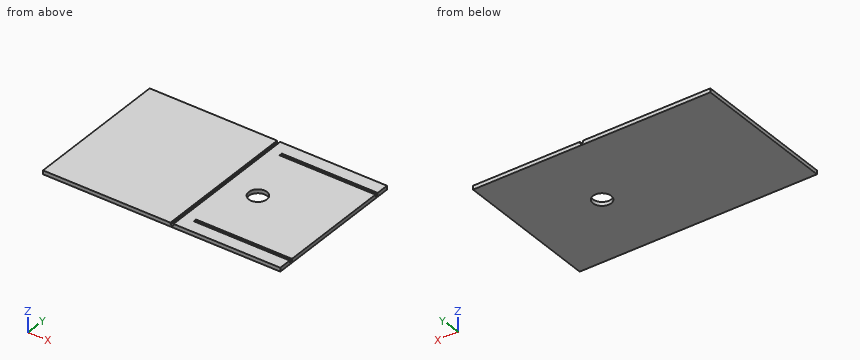
```python
from build123d import *

# Parameters (mm, degrees)
F0_W     = 1300
F0_H     = 800
F1_DEPTH = 21
F2_W     = 17
F2_H     = 800
F2_W_2   = 525
F2_H_2   = 17
F3_DEPTH = 10.2
F4_R     = 50
F5_DEPTH = 25


with BuildPart() as f1:
    # F0 (on Top) → F1 (new body)
    with BuildSketch(Plane.XY):
        with Locations((650, 400)):
            Rectangle(F0_W, F0_H)
    extrude(amount=F1_DEPTH)

    # F2 (on face) → F3 (cut)
    with BuildSketch(Plane.XY.offset(21)):
        with Locations((706.5, 400)):
            Rectangle(F2_W, F2_H)
        with Locations((1037.5, 721.5)):
            Rectangle(F2_W_2, F2_H_2)
        with Locations((1037.5, 78.5)):
            Rectangle(F2_W_2, F2_H_2)
    extrude(amount=-F3_DEPTH, mode=Mode.SUBTRACT)

    # F4 (on face) → F5 (cut)
    with BuildSketch(Plane.XY.offset(21)):
        with Locations((885, 400)):
            Circle(F4_R)
    extrude(amount=-F5_DEPTH, mode=Mode.SUBTRACT)


solid = f1.part
```
The listing builds one solid part. Answer for the finished solid, in the listing's coordinates (mm). Round coordinates to 2 decimals unless told otherwise and drop trailing zeros. Order: outer loops, then holes, each group sorted by start corner. A loop starts at its lowest first (then second) coordinate and runs counter-clockwise, first axis right, second up. Notation, with made-up numbers: (-2.5, 82.25) -> (6.5, 82.25) arc R22 ccw to (6.5, 105.25) -> close; hole circle Ø7 at (11.25, -21.5). An arc over 180 degrees is marked (long way). Answer as CSV lines item,"result".
Q1. A cutting plane is placed at B-B on y = 400. Determine the outline of the cut face in (x, z), plus the area to 3 significant figures.
Computed values:
outline,"(0, 0) -> (835, 0) -> (835, 21) -> (715, 21) -> (715, 10.8) -> (698, 10.8) -> (698, 21) -> (0, 21) -> close; (935, 0) -> (1300, 0) -> (1300, 21) -> (935, 21) -> close"
area,"25,000 mm^2"
Q2. A cutting plane is placed at C-C on x = 912.5. Determine the outline of the cut face in (y, z), plus the area to 3 significant figures.
Computed values:
outline,"(0, 0) -> (358.24, 0) -> (358.24, 21) -> (87, 21) -> (87, 10.8) -> (70, 10.8) -> (70, 21) -> (0, 21) -> close; (441.76, 0) -> (800, 0) -> (800, 21) -> (730, 21) -> (730, 10.8) -> (713, 10.8) -> (713, 21) -> (441.76, 21) -> close"
area,"14,700 mm^2"
Q3. Given pin 1 (5 mm diameter, centred on x = 1133, y = 77, fed in from +Z); pin 2 (5 mm diameter, centred on y = 720.5, z = 18.5, fed in from +X), each flat-ended and moving along its own axis, determine where each tip first touches the part or whether it passes through.
Computed values:
pin 1,"stops at z = 10.8"
pin 2,"stops at x = 775"
Q4. A cutting plane is placed at D-D on x = 1065. Determine the outline of the cut face in (y, z), plus the area to 3 significant figures.
Computed values:
outline,"(0, 0) -> (800, 0) -> (800, 21) -> (730, 21) -> (730, 10.8) -> (713, 10.8) -> (713, 21) -> (87, 21) -> (87, 10.8) -> (70, 10.8) -> (70, 21) -> (0, 21) -> close"
area,"16,500 mm^2"
Q5. A cutting plane is placed at A-A on z = 17.5. Determine the outline of the cut face in (x, y), plus the area to 3 significant figures.
Computed values:
outline,"(0, 0) -> (698, 0) -> (698, 800) -> (0, 800) -> close; (715, 0) -> (1300, 0) -> (1300, 70) -> (775, 70) -> (775, 87) -> (1300, 87) -> (1300, 713) -> (775, 713) -> (775, 730) -> (1300, 730) -> (1300, 800) -> (715, 800) -> close; hole circle Ø100 at (885, 400)"
area,"1,000,000 mm^2"
Q6. Consider line 1 (Y direction, x = 885, z = 13.5); line 2 (Y direction, x = 1210, z = 12); line 3 (Y direction, x = 885, z = 6). Determine where each line is inside the solid, lowest interval first. Write a range as from..to.
Computed values:
line 1,"y = 0..70, 87..350, 450..713, 730..800"
line 2,"y = 0..70, 87..713, 730..800"
line 3,"y = 0..350, 450..800"
